The listing builds one solid part. Answer for the finished solid, in the listing's coordinates (mm). Face numbers are marked on the shaded views. A direction names the side the tool comes from. Round coordinates to 2 decimals unless told otherwise and drop trailing zeros. Write each loop counter-clockwise with the first axis right and the second up, starting at its lowest first coordinate (ties: lowest second). Pieces come first, ordered by that corner, then holes. Notation, with made-up numbers: M 53.25,15 L 94.25,15 A20 cw 94.25,44 Z; hole C 25.5,54 d8. An arc over 180 degrees is marked long. One line per item, written item: value. Start each with the question number.
(1) Section A-A (y = -66) is taken. Determine the outline of the cut face in (x, z).
(2) Section B-B (y = 3.5) is taken. Determine the outline of the cut face in (x, z), plus the area to 3 significant figures.
(3) For the marked faces 4, 5 and 6, determine the directions among +Z, -Z, +X, -X, +Y, -Y from which every point of the face is accessible in a straight line to the end or side of a thin tool.
(4) Given P1, Ø1.5, axis at x = -8.5, y = -63, coming from the +Z side; P2, Ø5, axis at y = -5, z = 7.5, coming from the -X side; P3, Ø1.2, axis at y = 23.94, z = 0, coming from the -X side; P4, Ø2, axis at x = 9.5, z = -0.5, coming from the +Y side, each flat-ended and moving along its own axis, determine where each tip first touches the part or whether it passes through.
(5) Consider probe 1 along Y at (x, z) = (-3.75, 0); probe 2 along Z at (x, y) = (-0.5, -3); probe 3 along X at (y, z) = (-9, 0). Determine where each line is inside the solid, lowest interval first.
(6) For a pull along Y with two mould halves and no side action, classify the marked faces 1, 2 and 3 as released by +Y, released by -Y, zero draft, split by the parting line, or undercut.
```python
from build123d import *

# Parameters (mm, degrees)
SKETCH2_R               = 2.83366024
BOSS_EXTRUDE1_DEPTH     = 45
BOSS_EXTRUDE2_DEPTH     = 5
FILLET1_R               = 2
FILLET2_R               = 2
CUT_EXTRUDE2_DEPTH      = 115
CUT_EXTRUDE2_DEPTH_BACK = 96
SKETCH5_R               = 1
SKETCH8_R               = 2
CUT_EXTRUDE3_DEPTH      = 93


with BuildPart() as part:
    # Sketch1 → Revolve7 (revolve)
    with BuildSketch(Plane.XY, mode=Mode.PRIVATE) as revolve7_sk:
        Polygon((0, 0), (0, 28.475188422), (-4.956233819, 28.475188422), (-9.912467638, 27.282021021), (-9.912467638, 19.643055135), (-5.183583994, 0), align=None)
        with BuildLine():
            Line((0, -25.281339493), (0, 0))
            Line((0, 0), (-5.183583994, 0))
            add(Edge.make_bspline(
                [(-5.183583994, 0), (-8.573978987, -1.188883935), (-14.492218072, -9.39255897), (-12.177190855, -19.84099189), (-9.91246763, -25.281339493)],
                knots=[0, 0, 0, 0, 0.353823056, 1, 1, 1, 1], degree=3))
            Line((-9.91246763, -25.281339493), (-4.956233811, -25.281339493))
            Line((-4.956233811, -25.281339493), (0, -25.281339493))
        make_face()
    revolve(revolve7_sk.sketch.rotate(Axis((0, 53.654641341, 0), (0, -1, 0)), 270), axis=Axis((0, 53.654641341, 0), (0, -1, 0)))

    # Sketch2 → Boss-Extrude1 (add)
    with BuildSketch(Plane.XZ.offset(25.281339493)):
        with Locations(Location((-6.497142555, 0, 0), (0, 0, 90))):
            Circle(SKETCH2_R)
        with Locations(Location((6.497142555, 0, 0), (0, 0, 90))):
            Circle(SKETCH2_R)
    extrude(amount=BOSS_EXTRUDE1_DEPTH)

    # Sketch3 → Boss-Extrude2 (add)
    with BuildSketch(Plane.XZ.offset(70.281339493)):
        with BuildLine():
            Line((-9.330802795, 0), (-10.560252354, 8.471200618))
            Line((-10.560252354, 8.471200618), (-6.497142555, 11.576029804))
            Line((-6.497142555, 11.576029804), (-2.434032757, 8.471200618))
            Line((-2.434032757, 8.471200618), (-3.663482316, 0))
            ThreePointArc((-3.663482316, 0), (-6.497142555, -2.83366024), (-9.330802795, 0))
        make_face()
        with BuildLine():
            Line((2.917036225, 8.367030218), (7.097906526, 11.311372086))
            Line((7.097906526, 11.311372086), (11.03709893, 8.050760378))
            Line((11.03709893, 8.050760378), (9.478884483, -0.366172191))
            ThreePointArc((9.478884483, -0.366172191), (6.537086047, -3.087400346), (3.815857893, -0.14560191))
            Line((3.815857893, -0.14560191), (2.917036225, 8.367030218))
        make_face()
    extrude(amount=BOSS_EXTRUDE2_DEPTH)

    # Fillet1
    fillet1_edges = [part.edges().sort_by_distance(p)[0] for p in [
        (-6.497142555, -72.781339493, 11.576029804),
        (7.097906526, -72.781339493, 11.311372086),
    ]]
    fillet(fillet1_edges, radius=FILLET1_R)

    # Fillet2
    fillet2_edges = [part.edges().sort_by_distance(p)[0] for p in [
        (-2.434032757, -72.781339493, 8.471200618),
        (-10.560252354, -72.781339493, 8.471200618),
        (11.03709893, -72.781339493, 8.050760378),
        (2.917036225, -72.781339493, 8.367030218),
    ]]
    fillet(fillet2_edges, radius=FILLET2_R)

    # Sketch5 → Cut-Extrude2 (cut, two sides: drawn at the far end of the back side and taken through both)
    with BuildSketch(Plane(origin=(0, 0, 0), x_dir=(0, 0, -1), z_dir=(1, 0, 0)).offset(-CUT_EXTRUDE2_DEPTH_BACK)):
        with Locations(Location((0, 23.936282306, 0), (0, 0, 180))):
            Circle(SKETCH5_R)
    extrude(amount=CUT_EXTRUDE2_DEPTH + CUT_EXTRUDE2_DEPTH_BACK, mode=Mode.SUBTRACT)

    # Sketch8 → Cut-Extrude3 (cut)
    with BuildSketch(Plane(origin=(0, 28.475188422, 0), x_dir=(1, 0, 0), z_dir=(0, 1, 0))):
        with Locations(Location((0, 0, 0), (0, 0, 270))):
            Circle(SKETCH8_R)
    extrude(amount=-CUT_EXTRUDE3_DEPTH, mode=Mode.SUBTRACT)


solid = part.part
```
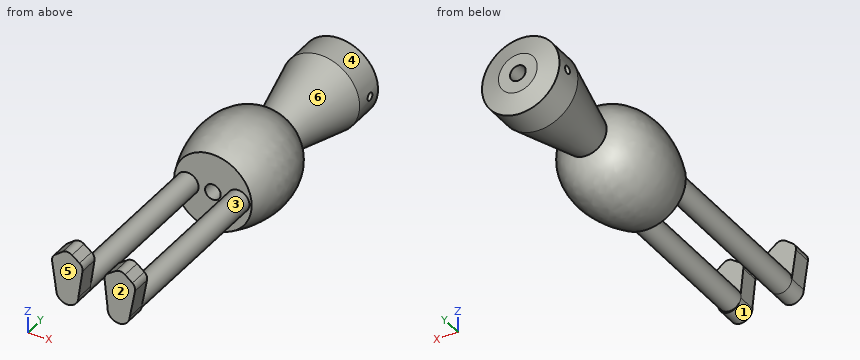
Recorded:
1. outline: C -6.5,0 d5.67; C 6.5,0 d5.67
2. outline: C 0,0 d12.05; hole C 0,0 d4
2. area: 102 mm2
3. face 4: +Y
3. face 5: +Z, -Z, +X, -X, -Y
3. face 6: none
4. P1: stops at z = 2.54
4. P2: stops at x = -10.04
4. P3: passes through
4. P4: stops at y = 27.62
5. probe 1: y = -75.28 to 22.94, 24.94 to 28.48
5. probe 2: z = -9.41 to -1.94, 1.94 to 9.41
5. probe 3: x = -12.2 to -2, 2 to 12.2
6. face 1: zero draft
6. face 2: released by -Y
6. face 3: undercut
